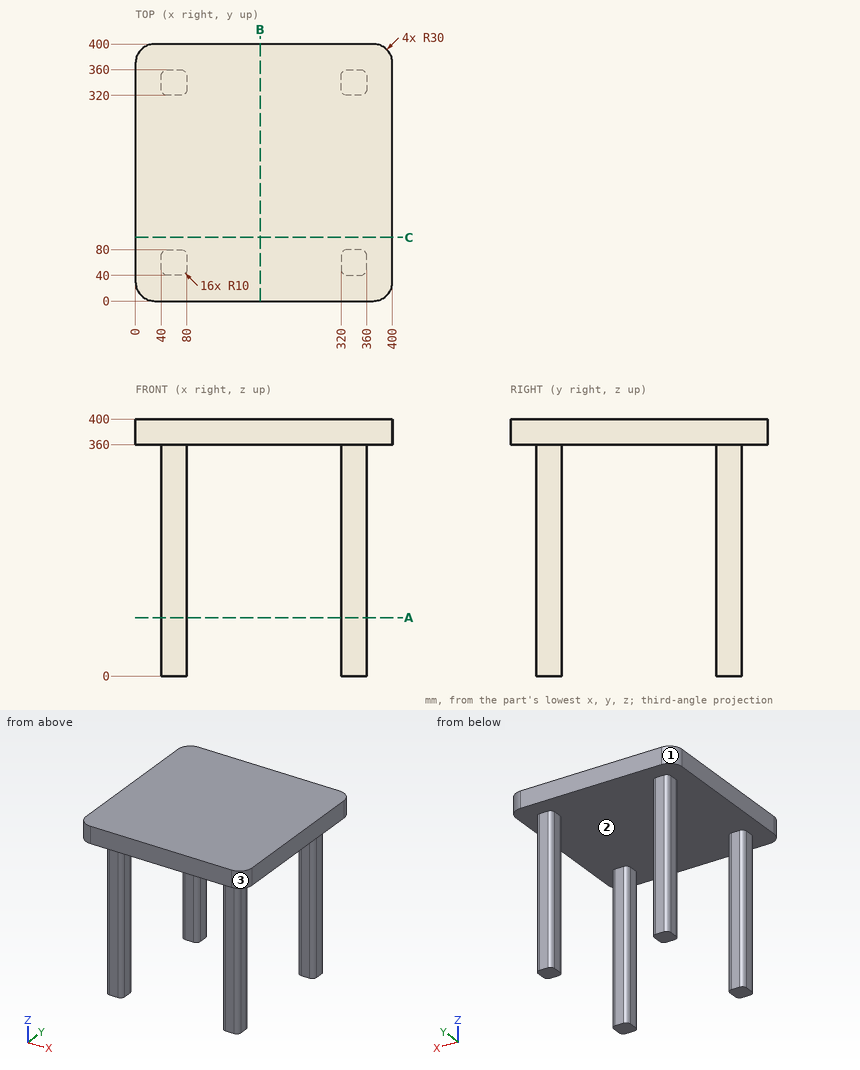
Design review of the part shown in the three views and the two pictorial views. Dimensions are in mm from the part's minimum x, y and z. Round coordinates to 2 decimals unless told otherwise and drop trailing zeros. Write each loop counter-clockwise with the first axis right and the second up, starting at its lowest first coordinate (ties: lowest second). Pieces come first, ordered by that corner, then holes. Notation, with made-up numbers: (-33, -31.5) - (22, -31.5) arc R25 ccw to (22, -1.5) - close; hole circle Ø8 at (49, 11). An arc over 180 degrees is marked (long way). Write item = value, one per line. Start each with the question number.
1. Wall thickness on L1, parallel to X at y = 51, z = 231.5; L2, parallel to Y at x = 48.5, z = 129.5: over which ranges is each line inside the solid? List them lowest first.
2. Consider section A-A on z = 91. Give the number of separate pieces and of enclosed holes in the cut face, plus the area to 3 significant figures.
3. Consider section B-B on x = 194. State the section outline as (y, z) points, plus the area to 3 significant figures.
4. Draft analysis for pull direction X (two halves, no side actions). For the marked faces 1, 2 and 3, state which applies: released by +X, released by -X, zero draft, split by the parting line, or undercut.
5. For pin 1 Ø16 at (x, z) = (337.5, 123) entering from -Y; pin 2 Ø6 at (y, z) = (344.5, 215) entering from +X; pin 3 Ø10 at (y, z) = (343, 246.5) entering from -X, all flat-tipped, find the tip position at first contact; note any pin that passes through.
Evaluation:
q1.L1 = 40 to 80, 320 to 360
q1.L2 = 40.11 to 79.89, 320.11 to 359.89
q2.separate_pieces = 4
q2.enclosed_holes = 0
q2.area = 6,060 mm2
q3.outline = (0, 360) - (400, 360) - (400, 400) - (0, 400) - close
q3.area = 16,000 mm2
q4.face_1 = released by -X
q4.face_2 = undercut
q4.face_3 = released by +X
q5.pin_1 = 40
q5.pin_2 = 360
q5.pin_3 = 40
